Could you check a few things on this model? Use its own coordinates, in mm. Give positions to 0.01 mm unless a question says otherwise; leave off trailing zeros. Write each question's results on one line, items separated by ' | '. Start each with the question number.
(1) Suppose I cut it at A-A (x = -26.5). Count the separate pieces of the cut face and the enclosed holes in it, and give its area (3 significant figures).
(2) I need wall thicknesses on line 1 (Z direction, x = -10, y = 12); line 2 (Y direction, x = -19, z = 21); line 3 (Z direction, x = -12.75, y = 12.5). Which ranges of each line are inside material? Lowest first, please.
(3) For pin 1 (1.5 mm diameter, centred on x = -9.5, y = 17.5, fed in from +Z); pin 2 (2 mm diameter, centred on x = -16, y = -3, fed in from +Z); pin 3 (1 mm diameter, centred on x = -25.5, z = 24.5, fed in from +Y), each with a flat end and sliding along its axis, tell me the tip position at first contact or that it passes through.
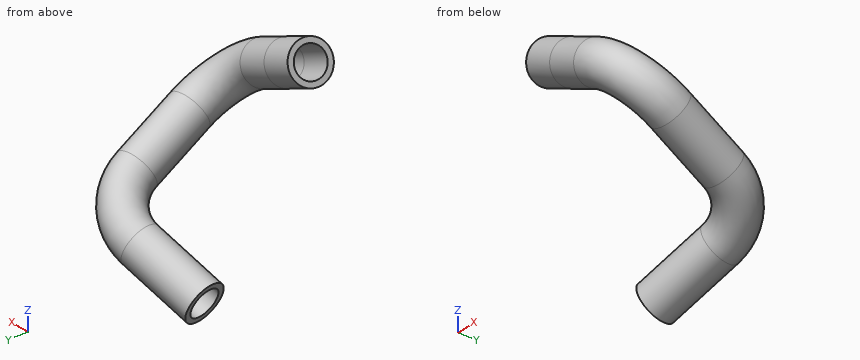
from build123d import *

# Parameters (mm, degrees)
SWEEP_SOTTILE1_PROFILE_R   = 3.175
SWEEP_SOTTILE1_PROFILE_R_2 = 2.325


with BuildPart() as part:
    # Sweep-Sottile1: sweep along a curve in space
    with BuildLine() as sweep_sottile1_path:
        Line((-26.865462484, -1.319578805, 27.359243174), (-21.558279201, -2.134095351, 24.681488818))
        Line((-16.139402673, -2.965753945, 21.94737932), (-21.558279201, -2.134095351, 24.681488818))
        ThreePointArc((-16.139402673, -2.965753945, 21.94737932), (-11.292193729, -1.598909493, 18.374309487), (-9.716090498, 3.233926671, 14.868582806))
        Line((-10.669409144, 12.472501866, 10.493247115), (-9.716090498, 3.233926671, 14.868582806))
        ThreePointArc((-17.751858156, 18.020311785, 5.184019113), (-12.960366508, 16.725311229, 7.716153393), (-10.669409144, 12.472501866, 10.493247115))
        Line((-17.751858156, 18.020311785, 5.184019113), (-28.425545748, 16.930941853, 1.25655118))
    # Sweep-Sottile1 profile (on start of the path) → Sweep-Sottile1 (sweep)
    with BuildSketch(Plane(origin=(-26.865462484, -1.319578805, 27.359243174), x_dir=(0.45046243787724455, 0, 0.8927953808469719), z_dir=(0.8845305472584387, -0.13575275761311742, -0.44629239268345283))):
        Circle(SWEEP_SOTTILE1_PROFILE_R)
        Circle(SWEEP_SOTTILE1_PROFILE_R_2, mode=Mode.SUBTRACT)
    sweep(path=sweep_sottile1_path.line)


solid = part.part
Output values:
1) separate pieces: 2 | enclosed holes: 1 | area: 25.6 mm2
2) line 1: 7.3 to 8.27, 13.22 to 14.19 | line 2: -5.05 to -3.6, -1.74 to -0.3 | line 3: 7.46 to 9.07, 11.56 to 13.04
3) pin 1: z = 11.13 | pin 2: z = 25.92 | pin 3: y = 1.2
